from build123d import *

# Parameters (mm, degrees)
F_3_8_0_375_DIAMETER_HOLE1_D     = 9.525
F_3_8_0_375_DIAMETER_HOLE1_DEPTH = 95.25
F_3_8_0_375_DIAMETER_HOLE1_TIP   = 2.861598698


with BuildPart() as part:
    # Sketch1 → Revolve1 (revolve)
    with BuildSketch(Plane.XY):
        Polygon((0, 0), (0, -101.6), (-6.35, -101.6), (-6.35, -6.35), (-12.7, -6.35), (-12.7, 0), align=None)
    revolve(axis=Axis((0, 0, 0), (0, -1, 0)))

    # 3/8 (0.375) Diameter Hole1
    with Locations(Plane(origin=(0, 0, 0), x_dir=(1, 0, 0), z_dir=(0, 1, 0))):
        with Locations((0, 0)):
            Hole(F_3_8_0_375_DIAMETER_HOLE1_D / 2, depth=F_3_8_0_375_DIAMETER_HOLE1_DEPTH)
            with Locations((0, 0, -(F_3_8_0_375_DIAMETER_HOLE1_DEPTH + F_3_8_0_375_DIAMETER_HOLE1_TIP / 2))):  # 118° drill point
                Cone(0, F_3_8_0_375_DIAMETER_HOLE1_D / 2, F_3_8_0_375_DIAMETER_HOLE1_TIP, mode=Mode.SUBTRACT)


solid = part.part
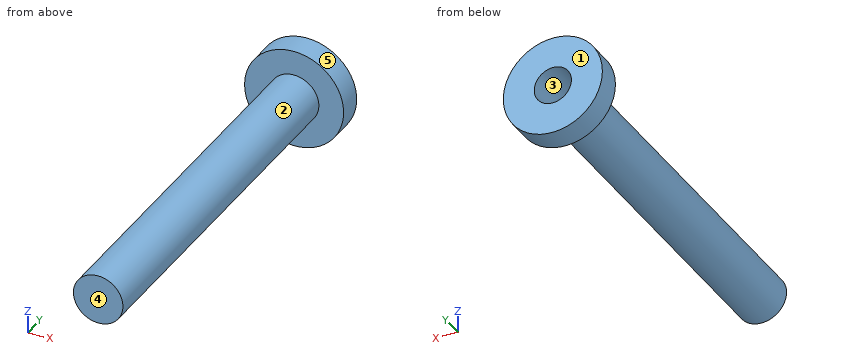
The listing builds one solid part. Answer for the finished solid, in the listing's coordinates (mm). Face numbers are marked on the shaded views. A direction names the side the tool comes from. Round coordinates to 2 decimals unless told otherwise and drop trailing zeros. Loops run counter-clockwise (first coordinate to the right, second up) from the corner with the lowest first, then second, coordinate; pieces in that order, holes last. Notation, with made-up numbers: M 57.25,40.25 L 61.25,40.25 A12 cw 61.25,52.25 Z; hole C 73.25,-16.5 d1. An arc over 180 degrees is marked long. Write each question's results on one line, items separated by ' | '. Start each with the question number.
1) Find section B-B on x = 7.5. Write down the section's boundary in (y, z).
2) Find section C-C on z = 8.75. Write down the section's boundary in (x, y), plus the area to 3 significant figures.
3) Straight lines are drawn through the part: probe 1 along Z at (x, y) = (0, -51); probe 2 along Y at (x, z) = (7.5, 9); probe 3 along X at (y, z) = (-38, -2.5). For each, find the intervals that lie inside material, in ascending order.
4) Determine the mould class of the marked faces 3, 4 and 5 for opening direction Z: pulls with the +Z half, pulls with the -Z half, needs draft (parallel to the pull), parting line crosses it, or undercut.
5) Which of the six approach directions +Z, -Z, +X, -X, +Y, -Y give full straight-line access (tool end or side, diameter ignored) to the marked faces 1 and 2?
6) Each of these flat-tipped pins is pushed along its axis until it touches: pin 1 (5 mm diameter, centred on x = -1, z = 9.5, fed in from -Y); pin 2 (4 mm diameter, centred on y = -54, z = 9.5, fed in from +X); pin 3 (8 mm diameter, centred on y = -38, z = 3, fed in from +X); pin 4 (1.5 mm diameter, centred on x = 4.5, y = -34, fed in from +Z). Where does it stop, or does it pass through?
Final values:
1) outline: M -6.35,-10.25 L 0,-10.25 L 0,10.25 L -6.35,10.25 Z
2) outline: M -9.2,-6.35 L 9.2,-6.35 L 9.2,0 L -9.2,0 Z | area: 117 mm²
3) probe 1: -6.35 to -4.76, 4.76 to 6.35 | probe 2: -6.35 to 0 | probe 3: -5.84 to -4.05, 4.05 to 5.84
4) face 3: undercut | face 4: needs draft | face 5: parting line crosses it
5) face 1: +Z, -Z, +X, -X, +Y | face 2: -Y
6) pin 1: y = -6.35 | pin 2: through | pin 3: x = 6.35 | pin 4: z = 5.12
